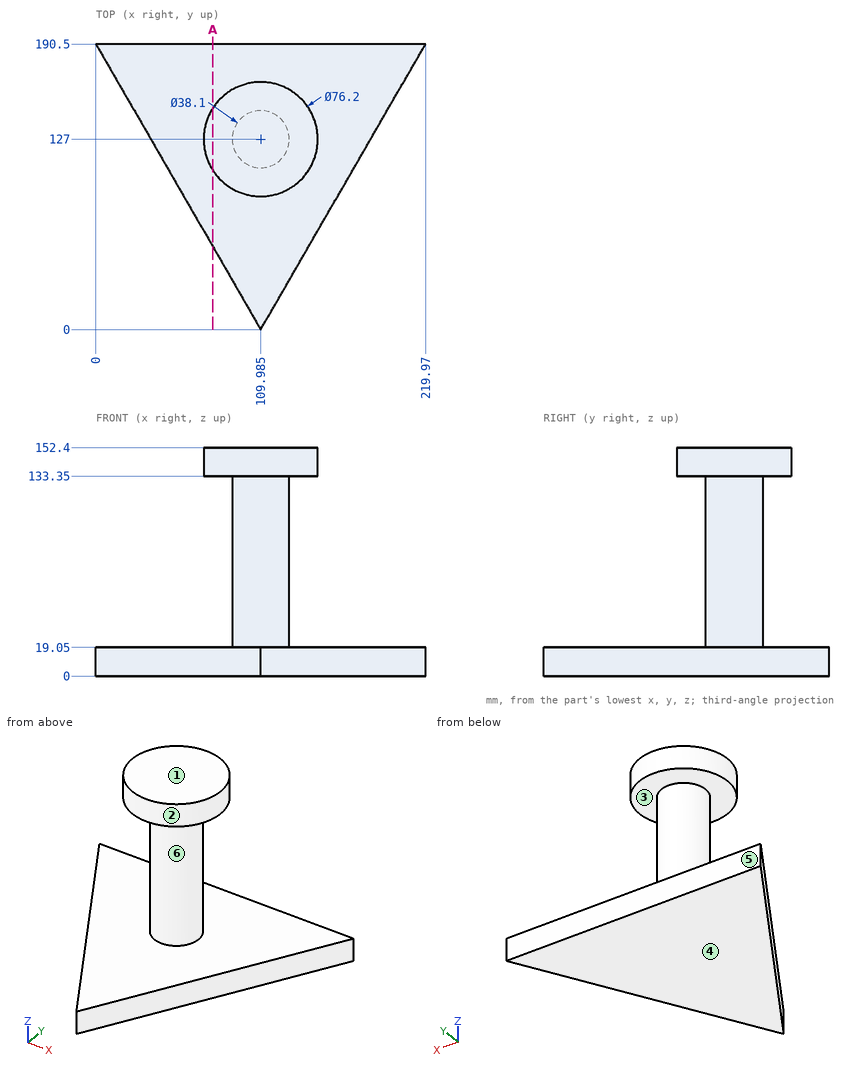
Geometry check sheet. Reference: drawing and pictorial views, mm from the part's lowest x, y, z. A direction names the side the tool comes from. Give positions to 0.01 mm unless a question says otherwise; leave off trailing zeros. Write each loop counter-clockwise with the first axis right and the second up, starting at its lowest first coordinate (ties: lowest second). Pieces come first, ordered by that corner, then holes. Notation, with made-up numbers: (53.25, 62.5) - (111.25, 62.5) arc R18 cw to (111.25, 80.5) - close; hole circle Ø7 at (63, 84.25). An arc over 180 degrees is marked (long way). Use a Markdown table: item, result.
Q1. Draft check along Z on the marked faces 4, 5 and 6. Enter one of: pulls with the +Z half, pulls with the -Z half, needs draft (parallel to the pull), parting line crosses it, or undercut.
Computed:
| item | result |
|---|---|
| face 4 | pulls with the -Z half |
| face 5 | needs draft |
| face 6 | undercut |
Q2. Thickness scan on L1, parallel to Z at x = 68.5, y = 123.5; L2, parallel to Z at x = 110.5, y = 147; L3, parallel to X at y = 17, z = 11.5. Record the ranges inside material, lowest first. Write a range as [from, to].
Computed:
| item | result |
|---|---|
| L1 | z = [0, 19.05] |
| L2 | z = [0, 19.05], [133.35, 152.4] |
| L3 | x = [100.17, 119.8] |
Q3. Set-up check for the marked faces 1, 2 and 3: record each of +Z, -Z, +X, -X, +Y, -Y from which the full face is reachable in a straight line by a thin tool's end or side.
Computed:
| item | result |
|---|---|
| face 1 | +Z, +X, -X, +Y, -Y |
| face 2 | +Z |
| face 3 | none |
Q4. Section check A-A, the plane x = 78. Enter the section's corners in (y, z), then the cut area to 3 significant figures.
Computed:
| item | result |
|---|---|
| outline | (55.4, 0) - (190.5, 0) - (190.5, 19.05) - (55.4, 19.05) - close; (106.3, 133.35) - (147.7, 133.35) - (147.7, 152.4) - (106.3, 152.4) - close |
| area | 3,360 mm² |
Q5. Go/stop test with flat-tipped pins: P1, Ø2, axis at x = 88, z = 44.5, coming from the -Y side; P2, Ø8, axis at y = 121.5, z = 95, coming from the -X side; P3, Ø3, axis at x = 97, z = 128, coming from the -Y side; P4, Ø2, axis at x = 114, z = 84, coming from the -Y side. Record where each tip stops, or that it passes through.
Computed:
| item | result |
|---|---|
| P1 | passes through |
| P2 | stops at x = 90.99 |
| P3 | stops at y = 111.8 |
| P4 | stops at y = 108.19 |
